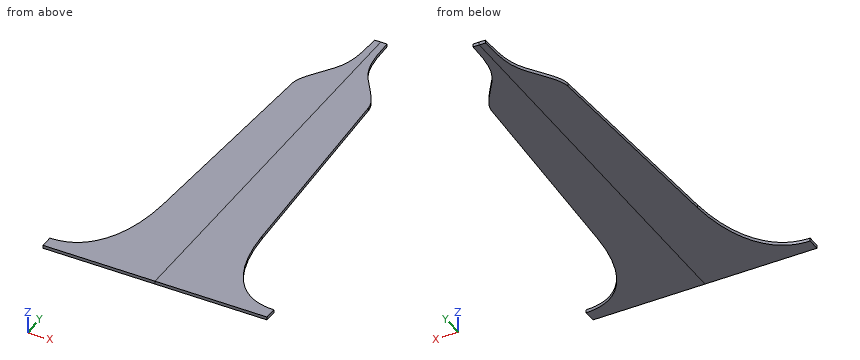
Autodesk Inventor part; units mm, degrees
ref_plane "YZ Plane" through (0, 0, 0) normal (1, 0, 0) x (0, 1, 0)
ref_plane "XZ Plane" through (0, 0, 0) normal (0, 1, 0) x (-1, 0, 0)
ref_plane "XY Plane" through (0, 0, 0) normal (0, 0, 1) x (1, 0, 0)
sketch "Sketch1" plane through (0, 0, 0) normal (0, 0, 1) x (1, 0, 0)
  line L0 (76.2, -12.7) -> (381, -12.7) construction
  line L1 (-76.2, -12.7) -> (-381, -12.7) construction
  line L2 (-76.2, 0) -> (-381, 0) construction
  line L3 (76.2, 0) -> (381, 0) construction
  line L4 (0, -116.2267) -> (0, 608.4603)
  line L5 (0, -12.7) -> (-114.3, -12.7)
  line L6 (-114.3, -12.7) -> (-114.3, 0)
  line L7 (0, 406.4) -> (-6.35, 406.4)
  line L8 (-39.0138, 312.42) -> (-50.5988, 93.6374)
  line L9 (39.0138, 312.42) -> (50.5988, 93.6374)
  line L10 (0, 406.4) -> (6.35, 406.4)
  line L11 (0, -12.7) -> (114.3, -12.7)
  line L12 (114.3, -12.7) -> (114.3, 0)
  spline S0 degree 4 poles (-6.35, 406.4) (-6.35, 381.154) (-10.7035, 365.7003) (-9.9482, 354.3709) (-38.2791, 326.2946) (-39.0138, 312.42) knots 0 0 0 0 0 0.492384 1 1 1 1 1
  line L13 (-6.35, 441.1174) -> (-6.35, 371.6826) construction
  arc A0 (-7.3193, 378.694) -> (-7.3193, 434.106) centre (-402.7904, 406.4) ccw construction
  spline S1 degree 4 poles (6.35, 406.4) (6.35, 381.154) (10.7035, 365.7003) (9.9482, 354.3709) (38.2791, 326.2946) (39.0138, 312.42) knots 0 0 0 0 0 0.492384 1 1 1 1 1
  line L14 (6.35, 441.1174) -> (6.35, 371.6826) construction
  arc A1 (7.3193, 434.106) -> (7.3193, 378.694) centre (402.7904, 406.4) ccw construction
  line L15 (-8.1247, 369.9755) -> (-17.7136, 348.6922) construction
  arc A2 (-17.4133, 351.2643) -> (-9.8522, 368.0464) centre (-62.6107, 381.7218) ccw construction
  line L16 (8.1247, 369.9755) -> (17.7136, 348.6922) construction
  arc A3 (9.8522, 368.0464) -> (17.4133, 351.2643) centre (62.6107, 381.7218) ccw construction
  spline S2 degree 3 poles (-50.5988, 93.6374) (-52.7393, 53.2143) (-67.314, 0) (-114.3, 0) knots 0 0 0 0 1 1 1 1
  line L17 (-100.9407, 0) -> (-127.6593, 0) construction
  arc A4 (-124.8332, 0.8979) -> (-103.7668, 0.8979) centre (-114.3, 62.2299) ccw construction
  spline S3 degree 3 poles (50.5988, 93.6374) (52.7393, 53.2143) (67.314, 0) (114.3, 0) knots 0 0 0 0 1 1 1 1
  line L18 (100.9407, 0) -> (127.6593, 0) construction
  arc A5 (103.7668, 0.8979) -> (124.8332, 0.8979) centre (114.3, 62.2299) ccw construction
  point P0 (0, 0)
  point P1 (-12.9192, 359.3339)
  point P2 (12.9192, 359.3339)
  dimension "d3" = 114.3
  dimension "d5" = 0.7
  dimension "d6" = 0.7
  dimension "d7" = 93.98
  dimension "d8" = 12.7
  dimension "d9" = 419.1
extrude "Extrusion1" add sketch "Sketch1" against normal blind 3.175
sketch "Etching" plane through (0, 0, 0) normal (0, 0, 1) x (1, 0, 0)
  line L0 (-114.3, -12.7) -> (114.3, -12.7)
  line L1 (114.3, -12.7) -> (114.3, 0)
  line L2 (50.5988, 93.6374) -> (39.0138, 312.42)
  line L3 (6.35, 406.4) -> (-6.35, 406.4)
  line L4 (-39.0138, 312.42) -> (-50.5988, 93.6374)
  line L5 (-114.3, 0) -> (-114.3, -12.7)
  line L6 (-45.7985, 184.2911) -> (45.7985, 184.2911)
  line L7 (0, -12.7) -> (0, 406.4)
  circle A0 centre (0, 184.2911) radius 5.08
  line L8 (-47.625, 12.7) -> (47.625, 12.7)
  line L9 (-47.625, 0) -> (-47.625, 12.7)
  line L10 (47.625, 12.7) -> (47.625, 0)
  line L11 (-114.3, 0) -> (114.3, 0)
  line L12 (37.9166, 92.9659) -> (29.8579, 245.1527)
  line L13 (42.5402, 245.8242) -> (29.8579, 245.1527)
  line L14 (37.9166, 92.9659) -> (50.5988, 93.6374)
  line L15 (-50.5988, 93.6374) -> (-37.9166, 92.9659)
  line L16 (-37.9166, 92.9659) -> (-29.8579, 245.1527)
  line L17 (-29.8579, 245.1527) -> (-42.5402, 245.8242)
  line L18 (-6.35, 298.8732) -> (6.35, 298.8732)
  line L19 (-6.35, 298.8732) -> (-6.35, 406.4)
  line L20 (6.35, 298.8732) -> (6.35, 406.4)
  dimension "d10" = 10.16
equation "\"d5\" = d6"
properties part number "Bottom Plate v2" material "Wood (Cherry)"
Check sheet for the modelled part. Datum: model origin and axes. Units: mm. Coordinates: 2 decimals unless noted, no trailing zeros. Write each loop counter-clockwise with the first axis right and the second up, starting at its lowest first coordinate (ties: lowest second). Pieces come first, ordered by that corner, then holes. Notation, with made-up numbers: M -35,-3 L -27,-3 A23 cw -27,13 Z; hole C 65.5,18 d7. An arc over 180 degrees is marked long. Answer as CSV lines item,"result".
Q1. Go/stop test with a flat-tipped pin: pin 1 (1 mm diameter, centred on y = 262, z = -2.5, fed in from -X). Record where the tip stops, or that it passes through.
Check result:
pin 1,"x = -41.71"
Q2. Cross-section at B-B (y = 198.5). Record the boundary of the cut face in (x, z) (3 decimals), then the cut area to 3 significant figures.
Check result:
outline,"M -45.046,-3.175 L 45.046,-3.175 L 45.046,0 L -45.046,0 Z"
area,"286 mm^2"
Q3. Cross-section at A-A (y = 110). Record the boundary of the cut face in (x, z) (3 decimals).
Check result:
outline,"M -49.732,-3.175 L 49.732,-3.175 L 49.732,0 L -49.732,0 Z"
Q4. Material ranges on probe 1 along X at (y, z) = (93, -2.7); probe 2 along X at (y, z) = (340, -2.75); probe 3 along Y at (x, z) = (72, -1.1), recorded low to high. Write a range as from..to.
Check result:
probe 1,"-50.63..50.63"
probe 2,"-25.21..25.21"
probe 3,"-12.7..21.58"
